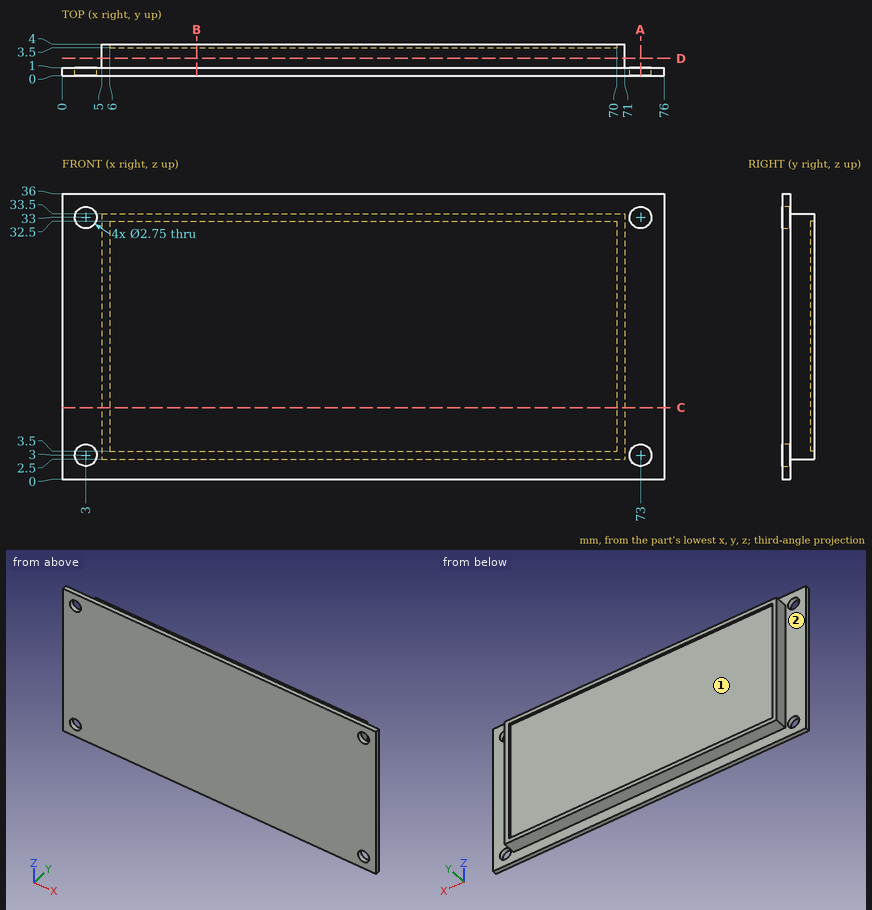
Check sheet for the drawn part. Datum: minimum x, y, z corner. Units: mm. Coordinates: 2 decimals unless noted, no trailing zeros. Loops run counter-clockwise (first coordinate to the right, second up) from the corner with the lowest first, then second, coordinate; pieces in that order, holes last. Notation, with made-up numbers: (84.5, -14) -> (109.5, -14) arc R25 cw to (109.5, 3) -> close; hole circle Ø1 at (67.5, 71). An arc over 180 degrees is marked (long way). Answer as CSV lines item,"result".
1) Release check for a two-part mould opening along Z. For the marked faces 1 and 2 record: +Z half, -Z half, draft (parallel to the pull), parting line (faces both ways), or undercut.
Found:
face 1,"undercut"
face 2,"draft"
2) Cross-section at D-D, the plane y = 2.2. Record the cut outline in (x, z), then the cut area to 3 significant figures.
Found:
outline,"(5, 2.5) -> (71, 2.5) -> (71, 33.5) -> (5, 33.5) -> close"
area,"2,050 mm2"
3) Cross-section at A-A, the plane x = 73. Record the cut outline in (y, z) (3 decimals).
Found:
outline,"(0, 0) -> (1, 0) -> (1, 1.625) -> (0, 1.625) -> close; (0, 4.375) -> (1, 4.375) -> (1, 31.625) -> (0, 31.625) -> close; (0, 34.375) -> (1, 34.375) -> (1, 36) -> (0, 36) -> close"
4) Depth check by flat-ended pin: pin 1 (1.5 mm diameter, centred on x = 18.5, y = 3, fed in from -Z); pin 2 (1.5 mm diameter, centred on x = 28.5, z = 17, fed in from +Y); pin 3 (3 mm diameter, centred on x = 73, z = 33, fed in from +Y); pin 4 (1.6 mm diameter, centred on x = 3, z = 3, fed in from +Y). Enter the tip coordinate at first touch or a pass-through.
Found:
pin 1,"stops at z = 2.5"
pin 2,"stops at y = 3.5"
pin 3,"stops at y = 1"
pin 4,"passes through"
5) Cross-section at B-B, the plane x = 17. Record the cut outline in (y, z).
Found:
outline,"(0, 0) -> (1, 0) -> (1, 2.5) -> (4, 2.5) -> (4, 3.5) -> (3.5, 3.5) -> (3.5, 32.5) -> (4, 32.5) -> (4, 33.5) -> (1, 33.5) -> (1, 36) -> (0, 36) -> close"
6) Thickness scan on L1, parallel to X at y = 0.5, z = 33 (3 decimals); L2, parallel to Z at x = 73, y = 0.45 (3 decimals); L3, parallel to X at y = 3.8, z = 31.5. Record the ranges inside material, lowest first. Write a range as from..to.
Found:
L1,"x = 0..1.625, 4.375..71.625, 74.375..76"
L2,"z = 0..1.625, 4.375..31.625, 34.375..36"
L3,"x = 5..6, 70..71"
7) Cross-section at C-C, the plane z = 9. Record the cut outline in (x, y).
Found:
outline,"(0, 0) -> (76, 0) -> (76, 1) -> (71, 1) -> (71, 4) -> (70, 4) -> (70, 3.5) -> (6, 3.5) -> (6, 4) -> (5, 4) -> (5, 1) -> (0, 1) -> close"
